Can you work these out from the model? Positions are in its coordinate system, mm. A direction names the side the tool comes from. Give positions to 0.01 mm unless a question says otherwise; leave off trailing zeros. Order: outer loops, then holes, each group sorted by start corner. A loop starts at its lowest first (then second) coordinate and runs counter-clockwise, first axis right, second up. Notation, with made-up numbers: (1, -24.75) - (21, -24.75) arc R18 ccw to (21, -16.75) - close; hole circle Ø7 at (23, 11). An arc over 180 degrees is marked (long way). Use one line per item in the form item = value. Start each with the question number.
1) Suppose I cut it at A-A, the plane x = 132.5. Write out the boundary of the cut face in (y, z), and give its area (3 significant figures).
2) Please list where these lines run through material, in increasing order: probe 1 along Y at (x, z) = (54, 2.05); probe 2 along Y at (x, z) = (0, 2.1); probe 3 along Y at (x, z) = (302, 0.8).
3) Suppose I cut it at B-B, the plane z = 3. State how many separate pieces and enclosed holes the cut face has, and give its area (3 significant figures).
4) Suppose I cut it at C-C, the plane x = 215. Write out the boundary of the cut face in (y, z), and give its area (3 significant figures).
5) We'd pull the mould along Y, two halves only. Please class faces 3 (the flat face through (227, 1, 0)), 4 (the cylindrical face through (360.5, 19.8, 2)), 5 (the cylindrical face through (-19.127, 19.057, 1.972)): released by +Y, released by -Y, zero draft, split by the parting line, or undercut.
6) For pin 1 (2 mm diameter, centred on x = 51, z = 2, fed in from +Y); pin 2 (6.5 mm diameter, centred on x = -12.99, y = 7.5, fed in from +Z); pin 3 (2 mm diameter, centred on y = -17, z = 1, fed in from +X); pin 4 (2 mm diameter, centred on x = 306, z = 1.5, fed in from -Y), each with a flat end and sliding along its axis, tell me the tip position at first contact or that it passes through.
7) Which directions (+Z, -Z, +X, -X, +Y, -Y) give clear straight access to the entire face, cutting with the end or side of a thin tool? Please do faces 1 (the cylindrical face through (180.5, 20.2, 2)), 2 (the flat face through (24.65, 33.41, 1.97)).
```python
from build123d import *

# Parameters (mm, degrees)
SKETCH_1_R      = 2
SKETCH_1_R_2    = 2.05
SKETCH_1_R_3    = 5
SKETCH_1_R_4    = 1.5
SKETCH_1_W      = 8.2
SKETCH_1_H      = 2.2
EXTRUDE_1_DEPTH = 4


with BuildPart() as part:
    # 草图1 → 凸台-拉伸1 (new body)
    with BuildSketch(Plane.XY):
        with BuildLine():
            Line((0, 27), (50, 40))
            Line((50, 40), (200, 40))
            Line((200, 40), (350, 50))
            Line((350, 50), (425, 50))
            Line((425, 50), (432.177174038, 50))
            ThreePointArc((432.177174038, 50), (462.315665579, 34.04486642), (475.446907157, 2.573205287))
            Line((475.446907157, 2.573205287), (482.5, 0))
            Line((482.5, 0), (475.446907157, -2.572885974))
            ThreePointArc((475.446907157, -2.572885974), (462.321199465, -34.038799886), (432.193107325, -49.997710289))
            Line((432.193107325, -49.997710289), (425, -50))
            Line((425, -50), (350, -50))
            Line((350, -50), (200, -40))
            Line((200, -40), (50, -40))
            Line((50, -40), (0, -27))
            Line((0, -27), (-2.35435733, -26.897156013))
            ThreePointArc((-2.35435733, -26.897156013), (-18.941976287, -19.240621984), (-26.857038268, -2.774796472))
            Line((-26.857038268, -2.774796472), (-35, 0))
            Line((-35, 0), (-26.857038268, 2.774796472))
            ThreePointArc((-26.857038268, 2.774796472), (-18.941976287, 19.240621984), (-2.35435733, 26.897156013))
            Line((-2.35435733, 26.897156013), (0, 27))
        make_face()
        with Locations((0, -15)):
            Circle(SKETCH_1_R, mode=Mode.SUBTRACT)
        with Locations((-12.990381057, -7.5)):
            Circle(SKETCH_1_R, mode=Mode.SUBTRACT)
        with Locations((-12.990381057, 7.5)):
            Circle(SKETCH_1_R, mode=Mode.SUBTRACT)
        with Locations((0, 15)):
            Circle(SKETCH_1_R, mode=Mode.SUBTRACT)
        with Locations((12.990381057, 7.5)):
            Circle(SKETCH_1_R, mode=Mode.SUBTRACT)
        with Locations((12.990381057, -7.5)):
            Circle(SKETCH_1_R, mode=Mode.SUBTRACT)
        with Locations((13.53, 0)):
            Circle(SKETCH_1_R_2, mode=Mode.SUBTRACT)
        with Locations((-6.765, -11.717323713)):
            Circle(SKETCH_1_R_2, mode=Mode.SUBTRACT)
        with Locations((-6.765, 11.717323713)):
            Circle(SKETCH_1_R_2, mode=Mode.SUBTRACT)
        Circle(SKETCH_1_R_3, mode=Mode.SUBTRACT)
        with Locations((394.9479618, -30.0520382)):
            Circle(SKETCH_1_R, mode=Mode.SUBTRACT)
        with Locations((382.5, 0)):
            Circle(SKETCH_1_R, mode=Mode.SUBTRACT)
        with Locations((275, 0)):
            Circle(SKETCH_1_R_4, mode=Mode.SUBTRACT)
        with Locations((125, 0)):
            Circle(SKETCH_1_R_4, mode=Mode.SUBTRACT)
        with Locations((467.5, 0)):
            Circle(SKETCH_1_R, mode=Mode.SUBTRACT)
        with Locations((455.0520382, -30.0520382)):
            Circle(SKETCH_1_R, mode=Mode.SUBTRACT)
        with Locations((455.0520382, 30.0520382)):
            Circle(SKETCH_1_R, mode=Mode.SUBTRACT)
        with Locations((394.9479618, 30.0520382)):
            Circle(SKETCH_1_R, mode=Mode.SUBTRACT)
        with Locations((425, 42.502596008)):
            Circle(SKETCH_1_R, mode=Mode.SUBTRACT)
        with Locations((425, -42.502596008)):
            Circle(SKETCH_1_R, mode=Mode.SUBTRACT)
        with Locations((200, 0)):
            Rectangle(SKETCH_1_W, SKETCH_1_H, mode=Mode.SUBTRACT)
        with Locations((50, 0)):
            Rectangle(SKETCH_1_W, SKETCH_1_H, mode=Mode.SUBTRACT)
        with Locations((350, 0)):
            Rectangle(SKETCH_1_W, SKETCH_1_H, mode=Mode.SUBTRACT)
        with BuildLine():
            Line((50, 30.5), (170, 30.5))
            ThreePointArc((170, 30.5), (180.5, 20), (170, 9.5))
            Line((170, 9.5), (50, 9.5))
            ThreePointArc((50, 9.5), (39.5, 20), (50, 30.5))
        make_face(mode=Mode.SUBTRACT)
        with BuildLine():
            Line((350, 30.5), (230, 30.5))
            ThreePointArc((230, 30.5), (219.5, 20), (230, 9.5))
            Line((230, 9.5), (350, 9.5))
            ThreePointArc((350, 9.5), (360.5, 20), (350, 30.5))
        make_face(mode=Mode.SUBTRACT)
        with BuildLine():
            Line((50, -30.5), (170, -30.5))
            ThreePointArc((170, -30.5), (180.5, -20), (170, -9.5))
            Line((170, -9.5), (50, -9.5))
            ThreePointArc((50, -9.5), (39.5, -20), (50, -30.5))
        make_face(mode=Mode.SUBTRACT)
        with BuildLine():
            Line((350, -30.5), (230, -30.5))
            ThreePointArc((230, -30.5), (219.5, -20), (230, -9.5))
            Line((230, -9.5), (350, -9.5))
            ThreePointArc((350, -9.5), (360.5, -20), (350, -30.5))
        make_face(mode=Mode.SUBTRACT)
        with BuildLine():
            ThreePointArc((456.82141298, 21.671356116), (464.472060808, 16.350447926), (462.824918175, 7.178131028))
            ThreePointArc((462.824918175, 7.178131028), (463.499999997, 0.000487034), (462.825099773, -7.177174038))
            ThreePointArc((462.825099773, -7.177174038), (464.472474468, -16.34944926), (456.821961265, -21.670551014))
            ThreePointArc((456.821961265, -21.670551014), (446.106697854, -32.198715901), (432.178131028, -37.824918175))
            ThreePointArc((432.178131028, -37.824918175), (425.000487034, -38.499999997), (417.822825962, -37.825099773))
            ThreePointArc((417.822825962, -37.825099773), (408.65055074, -39.472474468), (403.329448986, -31.821961265))
            ThreePointArc((403.329448986, -31.821961265), (397.776733311, -27.223955458), (393.17858702, -21.671356116))
            ThreePointArc((393.17858702, -21.671356116), (385.527939192, -16.350447926), (387.175081825, -7.178131028))
            ThreePointArc((387.175081825, -7.178131028), (386.500000003, -0.000487034), (387.174900227, 7.177174038))
            ThreePointArc((387.174900227, 7.177174038), (385.527525532, 16.34944926), (393.178038735, 21.670551014))
            ThreePointArc((393.178038735, 21.670551014), (397.776044542, 27.223266689), (403.328643884, 31.82141298))
            ThreePointArc((403.328643884, 31.82141298), (408.649552074, 39.472060808), (417.821868972, 37.824918175))
            ThreePointArc((417.821868972, 37.824918175), (424.999512966, 38.499999997), (432.177174038, 37.825099773))
            ThreePointArc((432.177174038, 37.825099773), (446.105883206, 32.1992499), (456.82141298, 21.671356116))
        make_face(mode=Mode.SUBTRACT)
    extrude(amount=EXTRUDE_1_DEPTH)


solid = part.part
```
Result sheet:
q1.outline = (-40, 0) - (-30.5, 0) - (-30.5, 4) - (-40, 4) - close; (-9.5, 0) - (9.5, 0) - (9.5, 4) - (-9.5, 4) - close; (30.5, 0) - (40, 0) - (40, 4) - (30.5, 4) - close
q1.area = 152 mm²
q2.probe_1 = -40 to -30.5, -9.5 to -1.1, 1.1 to 9.5, 30.5 to 40
q2.probe_2 = -27 to -17, -13 to -5, 5 to 13, 17 to 27
q2.probe_3 = -46.8 to -30.5, -9.5 to 9.5, 30.5 to 46.8
q3.separate_pieces = 1
q3.enclosed_holes = 28
q3.area = 24,800 mm²
q4.outline = (-41, 0) - (41, 0) - (41, 4) - (-41, 4) - close
q4.area = 328 mm²
q5.face_3 = zero draft
q5.face_4 = undercut
q5.face_5 = released by +Y
q6.pin_1 = 40
q6.pin_2 = 4
q6.pin_3 = 472.91
q6.pin_4 = -47.13
q7.face_1 = +Z, -Z
q7.face_2 = +Z, -Z, -X, +Y
